from build123d import *

# Parameters (mm, degrees)
SKETCH4_R           = 2
SKETCH4_R_2         = 1.25
SKETCH4_R_3         = 5
SKETCH4_R_4         = 3.96875
BOSS_EXTRUDE2_DEPTH = 6.35
SKETCH33_R          = 5
SKETCH33_R_2        = 3.499999985
BOSS_EXTRUDE6_DEPTH = 3


with BuildPart() as part:
    # Sketch4 → Boss-Extrude2 (new body)
    # profile 1 of 2: a face of its own
    with BuildSketch(Plane(origin=(0, 0, 0), x_dir=(1, 0, 0), z_dir=(0, 1, 0))):
        with BuildLine():
            Line((21.46596982, -18.4375), (40.257702493, -18.4375))
            ThreePointArc((40.257702493, -18.4375), (41.776936446, -18.121498883), (43.044160097, -17.225913752))
            Line((43.044160097, -17.225913752), (46.444939319, -13.579024524))
            ThreePointArc((46.444939319, -13.579024524), (47.203372649, -12.376980446), (47.468481715, -10.980610773))
            Line((47.468481715, -10.980610773), (47.468481715, 8.985116992))
            ThreePointArc((47.468481715, 8.985116992), (47.868781798, 10.685130659), (48.985566477, 12.027918285))
            Line((48.985566477, 12.027918285), (54.680415238, 16.319294633))
            ThreePointArc((54.680415238, 16.319294633), (55.797199918, 17.662082259), (56.1975, 19.362095927))
            Line((56.1975, 19.362095927), (56.1975, 26.9875))
            ThreePointArc((56.1975, 26.9875), (55.081576836, 29.681576836), (52.3875, 30.7975))
            Line((52.3875, 30.7975), (-4.7625, 30.7975))
            ThreePointArc((-4.7625, 30.7975), (-7.456576836, 29.681576836), (-8.5725, 26.9875))
            Line((-8.5725, 26.9875), (-8.5725, 0.781747009))
            Line((-8.5725, 0.781747009), (-20.917416467, -12.27322702))
            ThreePointArc((-20.917416467, -12.27322702), (-21.4498857, -17.515316011), (-16.517810325, -19.369406885))
            Line((-16.517810325, -19.369406885), (9.346561417, -11.463733294))
            Line((9.346561417, -11.463733294), (21.46596982, -18.4375))
        make_face()
        with Locations(Location((-17.78, -15.24, 0), (0, 0, 270))):
            Circle(SKETCH4_R, mode=Mode.SUBTRACT)
        with Locations(Location((0, -10.5, 0), (0, 0, 270))):
            Circle(SKETCH4_R_2, mode=Mode.SUBTRACT)
        with Locations(Location((0, 0, 0), (0, 0, 270))):
            Circle(SKETCH4_R_3, mode=Mode.SUBTRACT)
        with Locations(Location((24.012521227, -14.703599027, 0), (0, 0, 270))):
            Circle(SKETCH4_R, mode=Mode.SUBTRACT)
        with Locations(Location((0, 10.5, 0), (0, 0, 270))):
            Circle(SKETCH4_R_2, mode=Mode.SUBTRACT)
        with Locations(Location((-1.5875, 21.9075, 0), (0, 0, 270))):
            Circle(SKETCH4_R_4, mode=Mode.SUBTRACT)
        with Locations(Location((49.2125, 21.9075, 0), (0, 0, 270))):
            Circle(SKETCH4_R_4, mode=Mode.SUBTRACT)
    # profile 2 of 2: a face of its own
    with BuildSketch(Plane(origin=(0, 0, 0), x_dir=(1, 0, 0), z_dir=(0, 1, 0))):
        with BuildLine():
            Line((21.46596982, -18.4375), (40.257702493, -18.4375))
            ThreePointArc((40.257702493, -18.4375), (41.776936446, -18.121498883), (43.044160097, -17.225913752))
            Line((43.044160097, -17.225913752), (46.444939319, -13.579024524))
            ThreePointArc((46.444939319, -13.579024524), (47.203372649, -12.376980446), (47.468481715, -10.980610773))
            Line((47.468481715, -10.980610773), (47.468481715, 8.985116992))
            ThreePointArc((47.468481715, 8.985116992), (47.868781798, 10.685130659), (48.985566477, 12.027918285))
            Line((48.985566477, 12.027918285), (54.680415238, 16.319294633))
            ThreePointArc((54.680415238, 16.319294633), (55.797199918, 17.662082259), (56.1975, 19.362095927))
            Line((56.1975, 19.362095927), (56.1975, 26.9875))
            ThreePointArc((56.1975, 26.9875), (55.081576836, 29.681576836), (52.3875, 30.7975))
            Line((52.3875, 30.7975), (-4.7625, 30.7975))
            ThreePointArc((-4.7625, 30.7975), (-7.456576836, 29.681576836), (-8.5725, 26.9875))
            Line((-8.5725, 26.9875), (-8.5725, 0.781747009))
            Line((-8.5725, 0.781747009), (-20.917416467, -12.27322702))
            ThreePointArc((-20.917416467, -12.27322702), (-21.4498857, -17.515316011), (-16.517810325, -19.369406885))
            Line((-16.517810325, -19.369406885), (9.346561417, -11.463733294))
            Line((9.346561417, -11.463733294), (21.46596982, -18.4375))
        make_face()
        with Locations(Location((-17.78, -15.24, 0), (0, 0, 270))):
            Circle(SKETCH4_R, mode=Mode.SUBTRACT)
        with Locations(Location((0, -10.5, 0), (0, 0, 270))):
            Circle(SKETCH4_R_2, mode=Mode.SUBTRACT)
        with Locations(Location((0, 0, 0), (0, 0, 270))):
            Circle(SKETCH4_R_3, mode=Mode.SUBTRACT)
        with Locations(Location((24.012521227, -14.703599027, 0), (0, 0, 270))):
            Circle(SKETCH4_R, mode=Mode.SUBTRACT)
        with Locations(Location((0, 10.5, 0), (0, 0, 270))):
            Circle(SKETCH4_R_2, mode=Mode.SUBTRACT)
        with Locations(Location((-1.5875, 21.9075, 0), (0, 0, 270))):
            Circle(SKETCH4_R_4, mode=Mode.SUBTRACT)
        with Locations(Location((49.2125, 21.9075, 0), (0, 0, 270))):
            Circle(SKETCH4_R_4, mode=Mode.SUBTRACT)
    extrude(amount=-BOSS_EXTRUDE2_DEPTH)

    # Sketch33 → Boss-Extrude6 (add)
    with BuildSketch(Plane(origin=(0, 0, 0), x_dir=(1, 0, 0), z_dir=(0, 1, 0))):
        with Locations(Location((0, 0, 0), (0, 0, 270))):
            Circle(SKETCH33_R)
        with Locations(Location((0, 0, 0), (0, 0, 270))):
            Circle(SKETCH33_R_2, mode=Mode.SUBTRACT)
    extrude(amount=-BOSS_EXTRUDE6_DEPTH)


solid = part.part
Can you work these out from the model? Positions are in its coordinate system, mm. A direction names the side the tool comes from. Round coordinates to 2 decimals unless told otherwise and drop trailing zeros. Order: outer loops, then holes, each group sorted by start corner. A loop starts at its lowest first (then second) coordinate and runs counter-clockwise, first axis right, second up. Notation, with made-up numbers: (-7, -26.5) -> (15, -26.5) arc R19 cw to (15, -2.5) -> close; hole circle Ø10 at (82, 76). An arc over 180 degrees is marked (long way). Write each question's results on one line, items separated by ' | '. Start each with the question number.
Item 1: Will these pins go through, and if not, where does the flat tip stop? pin 1 (12 mm diameter, centred on x = 21, z = -5.5, fed in from +Y); pin 2 (2 mm diameter, centred on x = 0, z = -10.5, fed in from +Y); pin 3 (3 mm diameter, centred on y = -2, z = -3, fed in from +X); pin 4 (2 mm diameter, centred on y = -3.5, z = -11, fed in from -X).
Item 2: If we section it at A-A, the plane z = -10.5: Write out the boundary of the cut face in (x, y).
Item 3: If we section it at C-C, the plane z = 15.5: Write out the boundary of the cut face in (x, y).
Item 4: Thinking about a two-plate mould opening in Z: for faces 1 (the cylindrical face through (0.05, -3.13, -11.75)), 2 (the cylindrical face through (1.095, -3.131, -24.833)), 3 (the flat face through (-8.572, -3, -14)), 4 (the cylindrical face through (55.786, -3.131, -17.64)), which applies, +Z half, -Z half, draft (parallel to the pull), parting line (faces both ways), or undercut?
Item 5: Please list where these lines run through material, in increasing order: L1, parallel to Z at x = 24, y = -0.25; L2, parallel to X at y = -4.5, z = -27; L3, parallel to X at y = -1.9, z = 0.
Item 6: If we section it at B-B, the plane x = 0: Write out the boundary of the cut face in (y, z), then the cut area to 3 significant figures.
Item 7: Which directions (+Z, -Z, +X, -X, +Y, -Y) give clear straight access to the entire face, cutting with the end or side of a thin tool? Please do faces 5 (the flat face through (31, -3, 18.438)), 6 (the cylindrical face through (3.47, -1.48, -0.46)).
Item 8: If we section it at D-D, the plane y = -4: Write out the boundary of the cut face in (x, z), then the cut area to 3 significant figures.
Results:
1) pin 1: stops at y = 0 | pin 2: passes through | pin 3: stops at x = 47.47 | pin 4: stops at x = -8.57
2) outline: (-8.57, -6.35) -> (-1.25, -6.35) -> (-1.25, 0) -> (-8.57, 0) -> close; (1.25, -6.35) -> (47.78, -6.35) -> (47.78, 0) -> (1.25, 0) -> close
3) outline: (-22.09, -6.35) -> (-19.76, -6.35) -> (-19.76, 0) -> (-22.09, 0) -> close; (-15.8, -6.35) -> (-3.86, -6.35) -> (-3.86, 0) -> (-15.8, 0) -> close; (16.36, -6.35) -> (22.18, -6.35) -> (22.18, 0) -> (16.36, 0) -> close; (25.85, -6.35) -> (44.65, -6.35) -> (44.65, 0) -> (25.85, 0) -> close
4) face 1: undercut | face 2: undercut | face 3: draft | face 4: +Z half
5) L1: z = -30.8 to 12.7, 16.7 to 18.44 | L2: x = -8.57 to 56.2 | L3: x = -9.31 to -3.5, 3.5 to 47.47
6) outline: (-6.35, -30.8) -> (0, -30.8) -> (0, -25.54) -> (-6.35, -25.54) -> close; (-6.35, -18.27) -> (0, -18.27) -> (0, -11.75) -> (-6.35, -11.75) -> close; (-6.35, -9.25) -> (0, -9.25) -> (0, -3.5) -> (-3, -3.5) -> (-3, -5) -> (-6.35, -5) -> close; (-6.35, 5) -> (-3, 5) -> (-3, 3.5) -> (0, 3.5) -> (0, 9.25) -> (-6.35, 9.25) -> close; (-6.35, 11.75) -> (0, 11.75) -> (0, 14.32) -> (-6.35, 14.32) -> close | area: 154 mm2
7) face 5: +Z, +X, +Y, -Y | face 6: +Y, -Y
8) outline: (-20.92, 12.27) -> (-8.57, -0.78) -> (-8.57, -26.99) arc R3.81 ccw to (-4.76, -30.8) -> (52.39, -30.8) arc R3.81 ccw to (56.2, -26.99) -> (56.2, -19.36) arc R3.81 ccw to (54.68, -16.32) -> (48.99, -12.03) arc R3.81 cw to (47.47, -8.99) -> (47.47, 10.98) arc R3.81 ccw to (46.44, 13.58) -> (43.04, 17.23) arc R3.81 ccw to (40.26, 18.44) -> (21.47, 18.44) -> (9.35, 11.46) -> (-16.52, 19.37) arc R4.32 ccw to start; hole circle Ø4 at (-17.78, 15.24); hole circle Ø7.94 at (-1.59, -21.91); hole circle Ø10 at (0, 0); hole circle Ø2.5 at (0, -10.5); hole circle Ø2.5 at (0, 10.5); hole circle Ø4 at (24.01, 14.7); hole circle Ø7.94 at (49.21, -21.91) | area: 2,710 mm2
